Source: CAD feature listing. Evaluate the final solid. Frame: model axes, mm. Face numbers are marked on the shaded views. Give positions to 0.01 mm unless a question says otherwise; leave off trailing zeros. Loops run counter-clockwise (first coordinate to the right, second up) from the corner with the lowest first, then second, coordinate; pieces in that order, holes last.
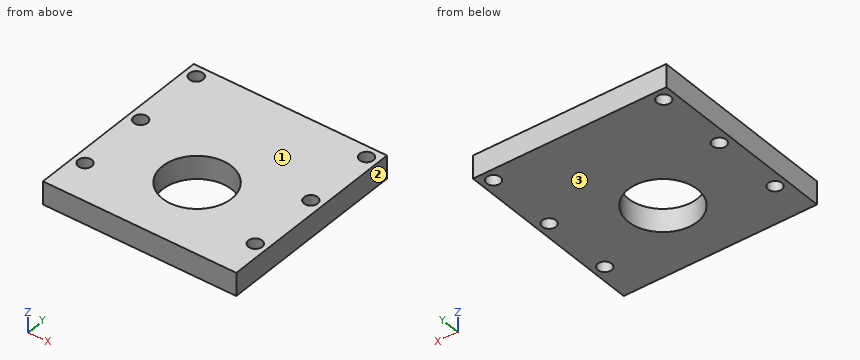
from build123d import *

# Parameters (mm, degrees)
SKETCH1_W                 = 53.34
SKETCH1_H                 = 53.34
BOSS_EXTRUDE1_DEPTH       = 6.35
SKETCH2_R                 = 9.525
CUT_EXTRUDE1_DEPTH        = 1
CUT_EXTRUDE1_DEPTH_BACK   = 7.35
F_6_CLEARANCE_HOLE1_D     = 3.7973
F_6_CLEARANCE_HOLE1_DEPTH = 6.35


with BuildPart() as part:
    # Sketch1 → Boss-Extrude1 (new body)
    with BuildSketch(Plane.XY):
        with Locations((26.67, 26.67)):
            Rectangle(SKETCH1_W, SKETCH1_H)
    extrude(amount=BOSS_EXTRUDE1_DEPTH)

    # Sketch2 → Cut-Extrude1 (cut, two sides)
    with BuildSketch(Plane.XY.offset(6.35)) as cut_extrude1_sk:
        with Locations((26.67, 20.32)):
            Circle(SKETCH2_R)
    extrude(amount=CUT_EXTRUDE1_DEPTH, mode=Mode.SUBTRACT)
    extrude(cut_extrude1_sk.sketch, amount=-CUT_EXTRUDE1_DEPTH_BACK, mode=Mode.SUBTRACT)

    # #6 Clearance Hole1
    with Locations(Plane.XY.offset(6.35)):
        with Locations((3.175, 50.165), (50.165, 50.165), (50.165, 10.795), (3.175, 10.795), (3.175, 30.48), (50.165, 30.48)):
            Hole(F_6_CLEARANCE_HOLE1_D / 2, depth=F_6_CLEARANCE_HOLE1_DEPTH)


solid = part.part
1) Cut plane D-D (z = 4). Return loops of the section in (x, y) (3 decimals).
Checks:
outline: (0, 0) - (53.34, 0) - (53.34, 53.34) - (0, 53.34) - close; hole circle Ø3.797 at (3.175, 10.795); hole circle Ø3.797 at (3.175, 30.48); hole circle Ø3.797 at (3.175, 50.165); hole circle Ø19.05 at (26.67, 20.32); hole circle Ø3.797 at (50.165, 10.795); hole circle Ø3.797 at (50.165, 30.48); hole circle Ø3.797 at (50.165, 50.165)
2) Cut plane B-B (y = 20.32). Return loops of the section in (x, z) (3 decimals).
Checks:
outline: (0, 0) - (17.145, 0) - (17.145, 6.35) - (0, 6.35) - close; (36.195, 0) - (53.34, 0) - (53.34, 6.35) - (36.195, 6.35) - close
3) Pull-direction query (Z, two-part tool) for the marked faces 1, 2 and 3; classes: released by +Z, released by -Z, zero draft, split by the parting line, or undercut.
Checks:
face 1: released by +Z
face 2: zero draft
face 3: released by -Z
4) Cut plane A-A (x = 26.67). Return loops of the section in (y, z) (3 decimals), and give its area (3 significant figures).
Checks:
outline: (0, 0) - (10.795, 0) - (10.795, 6.35) - (0, 6.35) - close; (29.845, 0) - (53.34, 0) - (53.34, 6.35) - (29.845, 6.35) - close
area: 218 mm2
5) Ray query, probe 1 along Y at (x, z) = (26.67, 5) (3 decimals); probe 2 along Y at (x, z) = (3, 2.25); probe 3 along X at (y, z) = (12, 1.5). Return the intervals inside material, ascending.
Checks:
probe 1: y = 0 to 10.795, 29.845 to 53.34
probe 2: y = 0 to 8.9, 12.69 to 28.59, 32.37 to 48.27, 52.06 to 53.34
probe 3: x = 0 to 1.71, 4.64 to 22.03, 31.31 to 48.7, 51.63 to 53.34
6) Contact query for a flat-ended pin moving along its axis: P1, Ø3, axis at x = 3.175, y = 50.165, coming from the -Z side. Output: stop coordinate, or through.
Checks:
P1: passes through
7) Cut plane C-C (y = 30.48). Return loops of the section in (x, z), and give its area (3 significant figures).
Checks:
outline: (0, 0) - (1.28, 0) - (1.28, 6.35) - (0, 6.35) - close; (5.07, 0) - (48.27, 0) - (48.27, 6.35) - (5.07, 6.35) - close; (52.06, 0) - (53.34, 0) - (53.34, 6.35) - (52.06, 6.35) - close
area: 290 mm2
